Check sheet for the modelled part. Datum: model origin and axes. Units: mm. A direction names the side the tool comes from. Give positions to 0.01 mm unless a question says otherwise; leave off trailing zeros. Order: outer loops, then holes, each group sorted by start corner. A loop starts at its lowest first (then second) coordinate and runs counter-clockwise, first axis right, second up. Notation, with made-up numbers: (-23, 31.5) - (22, 31.5) arc R10 ccw to (22, 50.5) - close; hole circle Ø4 at (44.25, -24). An arc over 180 degrees is marked (long way). Answer in a Markdown table with one row per item.
from build123d import *

# Parameters (mm, degrees)
SKETCH1_W           = 19
SKETCH1_H           = 35
BOSS_EXTRUDE1_DEPTH = 4
CUT_EXTRUDE1_DEPTH  = 21.310096012
BOSS_EXTRUDE2_DEPTH = 36
SKETCH4_R           = 2
CUT_EXTRUDE2_DEPTH  = 51.72266342
SKETCH5_R           = 2
CUT_EXTRUDE3_DEPTH  = 42.140004861


with BuildPart() as part:
    # Sketch1 → Boss-Extrude1 (new body)
    with BuildSketch(Plane(origin=(0, 0, 0), x_dir=(1, 0, 0), z_dir=(0, 1, 0))):
        Rectangle(SKETCH1_W, SKETCH1_H)
    extrude(amount=BOSS_EXTRUDE1_DEPTH)

    # Sketch2 → Cut-Extrude1 (cut, through all)
    with BuildSketch(Plane(origin=(0, 4, 0), x_dir=(1, 0, 0), z_dir=(0, 1, 0))):
        Polygon((9.5, 17.5), (-9.5, 7.81901646), (-9.5, 17.5), align=None)
    extrude(amount=-CUT_EXTRUDE1_DEPTH, mode=Mode.SUBTRACT)

    # Sketch3 → Boss-Extrude2 (add)
    with BuildSketch(Plane(origin=(0, 4, 0), x_dir=(1, 0, 0), z_dir=(0, 1, 0))):
        Polygon((9.5, 17.5), (-9.5, 7.81901646), (-9.5, 3.81901646), (9.5, 13.5), align=None)
    extrude(amount=BOSS_EXTRUDE2_DEPTH)

    # Sketch4 → Cut-Extrude2 (cut, through all)
    with BuildSketch(Plane(origin=(-5.120878649, 0, -10.050290234), x_dir=(-0.8910065241883689, 0, 0.45399049973954486), z_dir=(-0.4539904997395449, 0, -0.891006524188369))):
        with Locations((-11.409395725, 30)):
            Circle(SKETCH4_R)
        with Locations((-0.08519721, 20)):
            Circle(SKETCH4_R)
    extrude(amount=-CUT_EXTRUDE2_DEPTH, mode=Mode.SUBTRACT)

    # Sketch5 → Cut-Extrude3 (cut, through all)
    with BuildSketch(Plane(origin=(0, 4, 0), x_dir=(1, 0, 0), z_dir=(0, 1, 0))):
        with Locations(Location((-4.5, -7.5, 0), (0, 0, 270))):
            Circle(SKETCH5_R)
        with Locations(Location((4.5, -2.5, 0), (0, 0, 270))):
            Circle(SKETCH5_R)
    extrude(amount=-CUT_EXTRUDE3_DEPTH, mode=Mode.SUBTRACT)


solid = part.part
(1) Thickness scan on L1, parallel to X at y = 2, z = 2.5; L2, parallel to X at y = 1.5, z = 7.5; L3, parallel to Y at x = 1.75, z = -6.5. Record the ranges inside material, lowest first.
Geometry says:
| item | result |
|---|---|
| L1 | -9.5 to 2.5, 6.5 to 9.5 |
| L2 | -9.5 to -6.5, -2.5 to 9.5 |
| L3 | 0 to 4 |
(2) Access from +Z, -Z, +X, -X, +Y, -Y to the whole of each face (thin tool, end or side, straight path). Record for faces 1 (the flat face through (0, 4, 5)), 2 (the flat face through (9.5, 12, -14)).
Geometry says:
| item | result |
|---|---|
| face 1 | +Z, +X, +Y |
| face 2 | +Z, -Z, +X, +Y, -Y |
(3) Cross-section at B-B, the plane y = 30.5. Record the cut outline in (x, z), then the cut area to 3 significant figures.
Geometry says:
| item | result |
|---|---|
| outline | (-9.5, -7.82) - (3.32, -14.35) - (4.94, -11.18) - (-9.5, -3.82) - close; (6.77, -16.11) - (9.5, -17.5) - (9.5, -13.5) - (8.39, -12.93) - close |
| area | 62.2 mm² |
(4) Cross-section at C-C, the plane x = 2. Record the cut outline in (y, z).
Geometry says:
| item | result |
|---|---|
| outline | (0, -13.68) - (40, -13.68) - (40, -9.68) - (4, -9.68) - (4, 17.5) - (0, 17.5) - close |
(5) Cross-section at A-A, the plane z = 2.5. Record the cut outline in (x, y), then the cut area to 3 significant figures.
Geometry says:
| item | result |
|---|---|
| outline | (-9.5, 0) - (2.5, 0) - (2.5, 4) - (-9.5, 4) - close; (6.5, 0) - (9.5, 0) - (9.5, 4) - (6.5, 4) - close |
| area | 60.0 mm² |
(6) Gauge pin test, flat ends, axial feed: P1, Ø5, axis at x = 1.5, y = 13.5, coming from the -Z side; P2, Ø9.5, axis at x = 0, z = -0.5, coming from the +Y side; P3, Ø2, axis at x = -3.5, y = 11.5, coming from the -Z side. Record the tip position at first contact, or that the pin passes through.
Geometry says:
| item | result |
|---|---|
| P1 | z = -14.7 |
| P2 | y = 4 |
| P3 | z = -11.39 |
(7) Cross-section at D-D, the plane z = 13.5. Record the cut outline in (x, y).
Geometry says:
| item | result |
|---|---|
| outline | (-9.5, 0) - (9.5, 0) - (9.5, 4) - (-9.5, 4) - close |
(8) Mould release check, pull along Z, two halves, no side actions. Record for faces 3 (the flat face through (-0.133, 21.748, -8.592)), 4 (the cylindrical face through (-4.015, 21.983, -8.642)), 5 (the flat face through (0.133, 19.72, -12.727)), 6 (the cylindrical face through (-5.7, 2, 5.9)): pulls with the +Z half, pulls with the -Z half, needs draft (parallel to the pull), parting line crosses it, or undercut.
Geometry says:
| item | result |
|---|---|
| face 3 | pulls with the +Z half |
| face 4 | undercut |
| face 5 | pulls with the -Z half |
| face 6 | undercut |
